Build history of the part. All positions in model axes, mm. A direction names the side the tool comes from. Give positions to 0.01 mm unless a question says otherwise; leave off trailing zeros. Order: outer loops, then holes, each group sorted by start corner. A loop starts at its lowest first (then second) coordinate and runs counter-clockwise, first axis right, second up. Notation, with made-up numbers: M -27,38 L 28,38 A16 ccw 28,60 Z; hole C 0,37.5 d4. An arc over 180 degrees is marked long. Answer as CSV lines item,"result".
from build123d import *

# Parameters (mm, degrees)
SKIZZE2_W                       = 217
SKIZZE2_H                       = 155
AUFSATZ_LINEAR_AUSTRAGEN1_DEPTH = 20
WANDUNG1_T                      = -5
SCHNITT_LINEAR_AUSTRAGEN1_REACH = 192.256
SKIZZE7_R                       = 1.5
FASE1_SIZE                      = 3
SCHNITT_LINEAR_AUSTRAGEN2_DEPTH = 1


with BuildPart() as part:
    # Skizze2 → Aufsatz-Linear austragen1 (new body)
    with BuildSketch(Plane(origin=(0, 0, 0), x_dir=(1, 0, 0), z_dir=(0, 1, 0))):
        Rectangle(SKIZZE2_W, SKIZZE2_H)
    extrude(amount=AUFSATZ_LINEAR_AUSTRAGEN1_DEPTH)

    # Wandung1
    wandung1_openings = [part.faces().sort_by_distance(p)[0] for p in [
        (0, 20, 0),
    ]]
    offset(amount=WANDUNG1_T, openings=wandung1_openings, kind=Kind.INTERSECTION)

    # Skizze7 → Schnitt-Linear austragen1 (cut, up to next)
    with BuildSketch(Plane.XY.offset(77.5), mode=Mode.PRIVATE) as schnitt_linear_austragen1_sk1:
        with Locations((-93.5, 15)):
            Circle(SKIZZE7_R)
    schnitt_linear_austragen1_tool1 = extrude(schnitt_linear_austragen1_sk1.sketch, amount=-SCHNITT_LINEAR_AUSTRAGEN1_REACH, mode=Mode.PRIVATE) & part.part
    # Skizze7 → Schnitt-Linear austragen1 (cut, up to next)
    with BuildSketch(Plane.XY.offset(77.5), mode=Mode.PRIVATE) as schnitt_linear_austragen1_sk2:
        with Locations((-78.5, 15)):
            Circle(SKIZZE7_R)
    schnitt_linear_austragen1_tool2 = extrude(schnitt_linear_austragen1_sk2.sketch, amount=-SCHNITT_LINEAR_AUSTRAGEN1_REACH, mode=Mode.PRIVATE) & part.part
    # Skizze7 → Schnitt-Linear austragen1 (cut, up to next)
    with BuildSketch(Plane.XY.offset(77.5), mode=Mode.PRIVATE) as schnitt_linear_austragen1_sk3:
        with Locations((78.5, 15)):
            Circle(SKIZZE7_R)
    schnitt_linear_austragen1_tool3 = extrude(schnitt_linear_austragen1_sk3.sketch, amount=-SCHNITT_LINEAR_AUSTRAGEN1_REACH, mode=Mode.PRIVATE) & part.part
    # Skizze7 → Schnitt-Linear austragen1 (cut, up to next)
    with BuildSketch(Plane.XY.offset(77.5), mode=Mode.PRIVATE) as schnitt_linear_austragen1_sk4:
        with Locations((93.5, 15)):
            Circle(SKIZZE7_R)
    schnitt_linear_austragen1_tool4 = extrude(schnitt_linear_austragen1_sk4.sketch, amount=-SCHNITT_LINEAR_AUSTRAGEN1_REACH, mode=Mode.PRIVATE) & part.part
    add(schnitt_linear_austragen1_tool1.solids().sort_by_distance((-93.5, 15, 77.5))[0], mode=Mode.SUBTRACT)
    add(schnitt_linear_austragen1_tool2.solids().sort_by_distance((-78.5, 15, 77.5))[0], mode=Mode.SUBTRACT)
    add(schnitt_linear_austragen1_tool3.solids().sort_by_distance((78.5, 15, 77.5))[0], mode=Mode.SUBTRACT)
    add(schnitt_linear_austragen1_tool4.solids().sort_by_distance((93.5, 15, 77.5))[0], mode=Mode.SUBTRACT)

    # Fase1
    fase1_edges = [part.edges().sort_by_distance(p)[0] for p in [
        (0, 0, 77.5),
        (-108.5, 0, 0),
        (0, 0, -77.5),
        (108.5, 0, 0),
        (108.5, 10, 77.5),
        (-108.5, 10, 77.5),
        (-108.5, 10, -77.5),
        (108.5, 10, -77.5),
    ]]
    chamfer(fase1_edges, length=FASE1_SIZE)

    # Skizze8 → Schnitt-Linear austragen2 (cut)
    with BuildSketch(Plane.XZ):
        with BuildLine():
            Line((-96.881197846, -69.2), (-96.881197846, -62.8))
            ThreePointArc((-96.881197846, -62.8), (-96.969065812, -62.587867966), (-97.181197846, -62.5))
            Line((-97.181197846, -62.5), (-99.980384758, -62.5))
            ThreePointArc((-99.980384758, -62.5), (-100.240192379, -62.35), (-100.240192379, -62.05))
            Line((-100.240192379, -62.05), (-96.441005468, -55.469615242))
            ThreePointArc((-96.441005468, -55.469615242), (-96.103552133, -55.329837494), (-95.881197846, -55.619615242))
            Line((-95.881197846, -55.619615242), (-95.881197846, -61.2))
            ThreePointArc((-95.881197846, -61.2), (-95.793329881, -61.412132034), (-95.581197846, -61.5))
            Line((-95.581197846, -61.5), (-91.181197846, -61.5))
            ThreePointArc((-91.181197846, -61.5), (-90.969065812, -61.412132034), (-90.881197846, -61.2))
            Line((-90.881197846, -61.2), (-90.881197846, -54.8))
            ThreePointArc((-90.881197846, -54.8), (-90.793329881, -54.587867966), (-90.581197846, -54.5))
            Line((-90.581197846, -54.5), (-90.181197846, -54.5))
            ThreePointArc((-90.181197846, -54.5), (-89.969065812, -54.587867966), (-89.881197846, -54.8))
            Line((-89.881197846, -54.8), (-89.881197846, -61.2))
            ThreePointArc((-89.881197846, -61.2), (-89.793329881, -61.412132034), (-89.581197846, -61.5))
            Line((-89.581197846, -61.5), (-86.782010935, -61.5))
            ThreePointArc((-86.782010935, -61.5), (-86.522203314, -61.65), (-86.522203314, -61.95))
            Line((-86.522203314, -61.95), (-90.321390225, -68.530384758))
            ThreePointArc((-90.321390225, -68.530384758), (-90.65884356, -68.670162506), (-90.881197846, -68.380384758))
            Line((-90.881197846, -68.380384758), (-90.881197846, -62.8))
            ThreePointArc((-90.881197846, -62.8), (-90.969065812, -62.587867966), (-91.181197846, -62.5))
            Line((-91.181197846, -62.5), (-95.581197846, -62.5))
            ThreePointArc((-95.581197846, -62.5), (-95.793329881, -62.587867966), (-95.881197846, -62.8))
            Line((-95.881197846, -62.8), (-95.881197846, -69.2))
            ThreePointArc((-95.881197846, -69.2), (-95.969065812, -69.412132034), (-96.181197846, -69.5))
            Line((-96.181197846, -69.5), (-96.581197846, -69.5))
            ThreePointArc((-96.581197846, -69.5), (-96.793329881, -69.412132034), (-96.881197846, -69.2))
        make_face()
        with BuildLine():
            Line((-97.441005468, -59.20166605), (-98.508141571, -61.05))
            ThreePointArc((-98.508141571, -61.05), (-98.508141571, -61.35), (-98.24833395, -61.5))
            Line((-98.24833395, -61.5), (-97.181197846, -61.5))
            ThreePointArc((-97.181197846, -61.5), (-96.969065812, -61.412132034), (-96.881197846, -61.2))
            Line((-96.881197846, -61.2), (-96.881197846, -59.35166605))
            ThreePointArc((-96.881197846, -59.35166605), (-97.103552133, -59.061888302), (-97.441005468, -59.20166605))
        make_face(mode=Mode.SUBTRACT)
        with BuildLine():
            Line((-88.254254122, -62.95), (-89.321390225, -64.79833395))
            ThreePointArc((-89.321390225, -64.79833395), (-89.65884356, -64.938111698), (-89.881197846, -64.64833395))
            Line((-89.881197846, -64.64833395), (-89.881197846, -62.8))
            ThreePointArc((-89.881197846, -62.8), (-89.793329881, -62.587867966), (-89.581197846, -62.5))
            Line((-89.581197846, -62.5), (-88.514061743, -62.5))
            ThreePointArc((-88.514061743, -62.5), (-88.254254122, -62.65), (-88.254254122, -62.95))
        make_face(mode=Mode.SUBTRACT)
    extrude(amount=-SCHNITT_LINEAR_AUSTRAGEN2_DEPTH, mode=Mode.SUBTRACT)


solid = part.part
Item 1: Band-saw the part on C-C (x = 48.5). Give the cut face in (y, z), and give its area (3 significant figures).
Geometry says:
outline,"M 0,-74.5 L 3,-77.5 L 20,-77.5 L 20,-72.5 L 5,-72.5 L 5,72.5 L 20,72.5 L 20,77.5 L 3,77.5 L 0,74.5 Z"
area,"916 mm2"
Item 2: Band-saw the part on A-A (y = 10). Give the cut face in (x, z).
Geometry says:
outline,"M -108.5,-74.5 L -105.5,-77.5 L 105.5,-77.5 L 108.5,-74.5 L 108.5,74.5 L 105.5,77.5 L -105.5,77.5 L -108.5,74.5 Z; hole M -103.5,-72.5 L 103.5,-72.5 L 103.5,72.5 L -103.5,72.5 Z"
Item 3: Probe line 1 along Z through (x, y) = (45, 16.75); line 2 along X through (y, z) = (14.75, 24); line 3 along Y through (x, z) = (-12.5, -62.5). List the from-to ranges inside material, lowest first. Write a range as from..to.
Geometry says:
line 1,"z = -77.5..-72.5, 72.5..77.5"
line 2,"x = -108.5..-103.5, 103.5..108.5"
line 3,"y = 0..5"
Item 4: Drop flat-ended pins along their axis: pin 1 (2.5 mm diameter, centred on x = 78.5, y = 15, fed in from +Z); pin 2 (1.1 mm diameter, centred on y = 0.5, z = -65.5, fed in from +X); pin 3 (0.8 mm diameter, centred on x = -98.5, y = 0.5, fed in from +Z). Give the stop position or say it passes through.
Geometry says:
pin 1,"stops at z = -72.5"
pin 2,"stops at x = 106.55"
pin 3,"stops at z = 75.4"
Item 5: 3-axis set-ups, long thin cutter, end or side, ignore diameter. For faces 4 (the flat face through (-1, 12, 72.5)), 5 (the flat face through (-93, 1, -62)), 6 (the flat face through (-108.5, 11, 1)): which of +Z, -Z, +X, -X, +Y, -Y reach the whole face in a straight line?
Geometry says:
face 4,"+Y"
face 5,"-Y"
face 6,"+Z, -Z, -X, +Y, -Y"
Item 6: Pull direction X, two halves, no side cores. Call faces 1 (the flat face through (-1, 12, -72.5)), 2 (the flat face through (-1, 11, -77.5)), 3 (the flat face through (108.5, 11, 1)): released by +X, released by -X, zero draft, split by the parting line, or undercut.
Geometry says:
face 1,"undercut"
face 2,"zero draft"
face 3,"released by +X"
Item 7: Band-saw the part on B-B (z = -10.5). Give the cut face in (x, y), and give its area (3 significant figures).
Geometry says:
outline,"M -108.5,3 L -105.5,0 L 105.5,0 L 108.5,3 L 108.5,20 L 103.5,20 L 103.5,5 L -103.5,5 L -103.5,20 L -108.5,20 Z"
area,"1,230 mm2"
